Answer from the drawing. Dimensions are ordinates in mm from the lowest x, y and z of the part. A direction names the side the tool comes from. Round coordinates to 2 decimals unless told otherwise and drop trailing zeros. Loops run counter-clockwise (first coordinate to the right, second up) from the corner with the lowest first, then second, coordinate; pieces in that order, holes last.
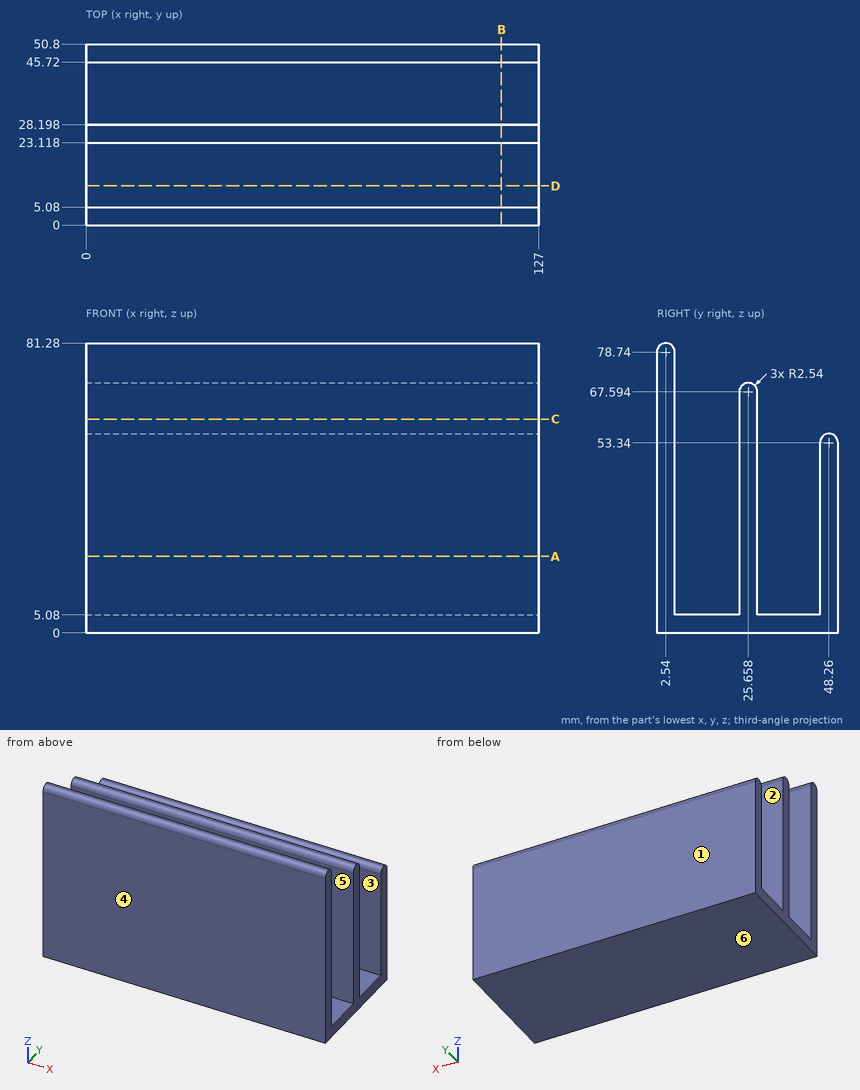
1. Which of the six approach directions +Z, -Z, +X, -X, +Y, -Y give full straight-line access (tool end or side, diameter ignored) to the marked faces 5 and 6?
Answer key:
face 5: +Z, +X, -X
face 6: -Z, +X, -X, +Y, -Y
2. Find section B-B (x = 116.5). Write down the section's boundary in (y, z), then the cut area to 3 significant figures.
Answer key:
outline: (0, 0) - (50.8, 0) - (50.8, 53.34) arc R2.54 ccw to (48.26, 55.88) arc R2.54 ccw to (45.72, 53.34) - (45.72, 5.08) - (28.2, 5.08) - (28.2, 67.59) arc R2.54 ccw to (25.66, 70.13) arc R2.54 ccw to (23.12, 67.59) - (23.12, 5.08) - (5.08, 5.08) - (5.08, 78.74) arc R2.54 ccw to (2.54, 81.28) arc R2.54 ccw to (0, 78.74) - close
area: 1,230 mm2
3. Consider probe 1 along Y at (x, z) = (26, 13); probe 2 along Y at (x, z) = (27, 57); probe 3 along Z at (x, y) = (33.5, 20). Determine where each line is inside the solid, lowest interval first.
Answer key:
probe 1: y = 0 to 5.08, 23.12 to 28.2, 45.72 to 50.8
probe 2: y = 0 to 5.08, 23.12 to 28.2
probe 3: z = 0 to 5.08
4. Given pin 1 (9 mm diameter, centred on x = 80, y = 39, fed in from +Z); pin 2 (3 mm diameter, centred on x = 111, z = 71, fed in from -Y); pin 3 (6 mm diameter, centred on x = 41.5, y = 45, fed in from +Z), each flat-ended and moving along its own axis, determine where each tip first touches the part or whether it passes through.
Answer key:
pin 1: stops at z = 5.08
pin 2: stops at y = 0
pin 3: stops at z = 55.87
5. Find section C-C (z = 60). Write down the section's boundary in (x, y).
Answer key:
outline: (0, 0) - (127, 0) - (127, 5.08) - (0, 5.08) - close; (0, 23.12) - (127, 23.12) - (127, 28.2) - (0, 28.2) - close
6. Determine the mould class of the marked faces 1, 2, 3 and 4 for opening direction Y: +Y half, -Y half, draft (parallel to the pull), parting line (faces both ways), or undercut.
Answer key:
face 1: +Y half
face 2: undercut
face 3: undercut
face 4: -Y half
7. Find section D-D (y = 11). Write down the section's boundary in (x, z).
Answer key:
outline: (0, 0) - (127, 0) - (127, 5.08) - (0, 5.08) - close
8. Find section A-A (z = 21.5). Write down the section's boundary in (x, y).
Answer key:
outline: (0, 0) - (127, 0) - (127, 5.08) - (0, 5.08) - close; (0, 23.12) - (127, 23.12) - (127, 28.2) - (0, 28.2) - close; (0, 45.72) - (127, 45.72) - (127, 50.8) - (0, 50.8) - close
